Autodesk Inventor part; units mm, degrees
ref_plane "YZ Plane" through (0, 0, 0) normal (1, 0, 0) x (0, 1, 0)
ref_plane "XZ Plane" through (0, 0, 0) normal (0, 1, 0) x (-1, 0, 0)
ref_plane "XY Plane" through (0, 0, 0) normal (0, 0, 1) x (1, 0, 0)
sketch "スケッチ1" plane through (0, 0, 0) normal (0, 1, 0) x (-1, 0, 0)
  circle A0 centre (0, 0) radius 1.15
  circle A1 centre (0, 0) radius 2
  circle A2 centre (0, 0) radius 3.5
  line L0 (0, 0) -> (0, 3.5)
  line L1 (2, 0) -> (-2, 0)
  line L2 (2, 0) -> (2, -2.8723)
  line L3 (-2, 0) -> (-2, -2.8723)
  line L4 (0, 2) -> (3.5, 2)
  line L5 (3.5, 2) -> (3.5, 6)
  line L6 (3.5, 6) -> (0, 6)
  line L7 (0, 6) -> (0, 2)
  line L8 (0, 6) -> (3.5, 6)
  line L9 (3.5, 6) -> (3.5, 0)
  line L10 (3.5, 0) -> (0, 0)
  line L11 (0, 0) -> (0, 6)
  line L12 (0, 0) -> (0, -8)
  line L13 (0, 0) -> (3.5, 0)
  line L14 (3.5, 0) -> (3.5, -8)
  line L15 (3.5, -8) -> (0, -8)
  line L16 (0, -8) -> (0, 0)
  line L17 (2, -2.8723) -> (2, -8)
  line L18 (0, -8) -> (3.5, -4.5)
  line L19 (0, -8) -> (4.9497, -8) construction
  line L20 (0, 0) -> (3.5, 0)
  line L21 (3.5, 0) -> (3.5, -9)
  line L22 (3.5, -9) -> (0, -9)
  line L23 (0, -9) -> (0, 0)
  line L24 (0, 2) -> (4, 2)
  line L25 (4, 2) -> (4, 9)
  line L26 (4, 9) -> (0, 9)
  line L27 (0, 9) -> (0, 2)
  line L28 (0, 9) -> (4, 9)
  line L29 (4, 9) -> (4, -9)
  line L30 (4, -9) -> (0, -9)
  line L31 (0, -9) -> (0, 9)
  line L32 (0, 0) -> (2, 0)
  line L33 (2, 0) -> (2, -9)
  line L34 (2, -9) -> (0, -9)
  line L35 (0, -9) -> (0, 0)
  point P0 (2, -6)
  point P1 (0, -3.5)
  dimension "d0" = 2.3
  dimension "d1" = 4
  dimension "d2" = 7
  dimension "d3" = 3.5
  dimension "d4" = 4
  dimension "d5" = 8
  dimension "d6" = 45
  dimension "d40" = 9
  dimension "d41" = 4
  dimension "d42" = 7
extrude "押し出し1" add sketch "スケッチ1" along normal blind 3 contours A1 L3 A2 L0
extrude "押し出し2" add sketch "スケッチ1" along normal blind 4.5 contours L10 A2 L2 | A1 L4 A2 L10 | L0 A2 L4 | A2 L14 L18 L17 | A2 L4 L9 | L9 L24 L29 L30 L21 L14 | L7 L6 L5 L4 A2 | L18 L14 L15 L17 | L5 L6 L27 L26 L25 L24 | L15 L21 L22 L33
extrude "押し出し3" add sketch "スケッチ1" against normal blind 1 contours L1 A1 L12 A0 | A0 L0 A1 L1 | A0 L1 A1 L0 | L12 A1 L1 A0 | L2 A2 L12 A1 | L10 A2 L2 | A1 L4 A2 L10 | A1 L3 A2 L0 | L0 A2 L4 | L12 A2 L3 A1 | L17 L18 L12 A2 | A2 L14 L18 L17 | A2 L4 L9 | L9 L24 L29 L30 L21 L14 | L7 L6 L5 L4 A2 | L18 L14 L15 L17 | L17 L15 L18 | L5 L6 L27 L26 L25 L24 | L15 L33 L22 L23 | L15 L21 L22 L33
sketch "スケッチ4" plane through (0, 4.5, 0) normal (0, 1, 0) x (1, 0, 0)
  circle A0 centre (0, 0) radius 1.15
  circle A1 centre (0, 0) radius 2
  circle A2 centre (0, 0) radius 3.5
  line L0 (-4, 9) -> (-4, -9)
  line L1 (0, 0) -> (-4, 0)
  line L2 (-4, 0) -> (-4, -9)
  line L3 (-4, -9) -> (0, -9)
  line L4 (0, -9) -> (0, 0)
  line L5 (0, 0) -> (-4, 0)
  line L6 (-4, 0) -> (-4, 9)
  line L7 (-4, 9) -> (0, 9)
  line L8 (0, 9) -> (0, 0)
  point P0 (0, -3.5)
  point P1 (0, 3.5)
  dimension "d43" = 2.3
  dimension "d44" = 4
  dimension "d45" = 7
  dimension "d46" = 4
  dimension "d47" = 9
extrude "押し出し6" add sketch "スケッチ4" along normal blind 1 contours A0 L8 A1 L4 | A0 L1 A1 L8 | L4 A1 L1 A0 | L8 A2 L4 A1 | A1 L1 A2 L8 | L4 A2 L1 A1 | A2 L1 L0 L7 L8 | L4 L3 L0 L1 A2
sketch "スケッチ5" plane through (-4, -1, 9) normal (0, 0, 1) x (1, 0, 0)
  line L0 (4, 0) -> (4, 4)
  line L1 (4, 0) -> (0, 0)
  line L2 (0, 0) -> (0, 1)
  line L3 (0, 1) -> (4, 1)
  line L4 (4, 1) -> (4, 0)
  line L5 (4, 1) -> (2.5, 1)
  line L6 (2.5, 1) -> (2.5, 1.5)
  line L7 (2.5, 1.5) -> (4, 1.5)
  line L8 (4, 1.5) -> (4, 1)
  line L9 (4, 6.5) -> (0, 6.5)
  line L10 (0, 6.5) -> (2, 6.5)
  line L11 (2, 6.5) -> (2, 4.25)
  line L12 (2, 4.25) -> (0, 4.25)
  line L13 (0, 4.25) -> (0, 6.5)
  circle A0 centre (2, 4.25) radius 1.1
  dimension "d50" = 4
  dimension "d51" = 1
  dimension "d52" = 1.5
  dimension "d53" = 0.5
  dimension "d54" = 2
  dimension "d55" = 2.25
  dimension "d56" = 2.2
extrude "押し出し7" cut sketch "スケッチ5" against normal blind 7 contours A0 L12 L11 | L11 L12 A0
hole "穴2" at (-1.5, 0.5, 9) direction (0, 0, -1) diameter 1 end through all
chamfer "面取り1" distance 0.5 angle 45 3 edges at (0, -1, 6.25) (0, 5.5, 6.25) (-4, 5.5, 0)
chamfer "面取り2" distance 1.5 angle 45 1 edges at (-4, -1, 0)
sketch "スケッチ6" plane through (0, 0, -9) normal (0, 0, -1) x (-1, 0, 0)
  line L0 (0, 5.5) -> (4, 5.5)
  line L1 (4, 5.5) -> (4, -1)
  line L2 (4, -1) -> (0, -1)
  line L3 (0, -1) -> (0, 5.5)
  point P0 (0, 0)
  dimension "d72" = 4
  dimension "d73" = 6.5
extrude "押し出し8" cut sketch "スケッチ6" against normal blind 1
properties part number "rod6.2"
For this review, take the finished solid that the model builds, in its own axes (mm). A direction names the side the tool comes from. Coordinates: 2 decimals unless noted, no trailing zeros. Order: outer loops, then holes, each group sorted by start corner. A loop starts at its lowest first (then second) coordinate and runs counter-clockwise, first axis right, second up. Notation, with made-up numbers: (4, 57.5) -> (17, 57.5) arc R22 cw to (17, 65.5) -> close; hole circle Ø6 at (68, -35.75). An arc over 180 degrees is marked (long way). Return JSON: item names as keys, results as strings.
1. Machinability: for faces 5 (the flat face through (-4, 3, 1)), 6 (the cylindrical face through (0, 2, 2)), 7 (the flat face through (0, 5, -6)), 8 (the cylindrical face through (-0.95, 3.58, 5.55)), which of the approach directions +Z, -Z, +X, -X, +Y, -Y give a long, thin tool a straight path to every point of the face, cutting with its end or side? Answer none if there is none.
Answer block:
{"face 5": "+Z, -Z, -X, +Y, -Y", "face 6": "-Z", "face 7": "-Z, +X, +Y, -Y", "face 8": "+Z"}
2. We need section D-D on z = 2.25. Write out the cut boundary in (x, y), and give its area (3 significant figures).
Answer block:
{"outline": "(-4, 0.5) -> (-2.5, -1) -> (2.68, -1) -> (2.68, 3) -> (0, 3) -> (0, 4.5) -> (2.68, 4.5) -> (2.68, 5.5) -> (-3.5, 5.5) -> (-4, 5) -> close; hole circle Ø2.2 at (-2, 3.25); hole circle Ø1 at (-1.5, 0.5)", "area": "33.6 mm²"}
3. We need section A-A on x = 3.25. Write out the cut boundary in (y, z).
Answer block:
{"outline": "(-1, -1.3) -> (3, -1.3) -> (3, 1.3) -> (-1, 1.3) -> close; (4.5, -1.3) -> (5.5, -1.3) -> (5.5, 1.3) -> (4.5, 1.3) -> close"}
4. We need section B-B on z = -0.5. Write out the cut boundary in (x, y), and give its area (3 significant figures).
Answer block:
{"outline": "(-4, 0.5) -> (-2.5, -1) -> (-1.04, -1) -> (-1.04, 0) -> (-2, 0) -> (-2, 4.5) -> (-1.04, 4.5) -> (-1.04, 5.5) -> (-3.5, 5.5) -> (-4, 5) -> close; (1.04, -1) -> (3.46, -1) -> (3.46, 3) -> (2, 3) -> (2, 0) -> (1.04, 0) -> close; (1.04, 4.5) -> (3.46, 4.5) -> (3.46, 5.5) -> (1.04, 5.5) -> close", "area": "22.9 mm²"}
5. For pin 1 Ø1.8 at (x, z) = (0, 0) entering from +Y; pin 2 Ø1.1 at (x, y) = (-2, 3) entering from +Z; pin 3 Ø0.5 at (y, z) = (5, -5) entering from +X; pin 4 Ø3 at (y, z) = (1.5, -3.5) entering from +X, all flat-tipped, find the tip position at first contact; note any pin that passes through.
Answer block:
{"pin 1": "through", "pin 2": "z = 2", "pin 3": "x = 0", "pin 4": "x = 2.87"}
6. For line 1 (Y direction, x = 3, z = 1.5); line 2 (Y direction, x = -1.5, z = 5.25); line 3 (Y direction, x = -1.5, z = -1.75), list the stretches that pass through material, from the lowest coordinate up. Write a range as from..to.
Answer block:
{"line 1": "-1..3, 4.5..5.5", "line 2": "-1..0, 1..2.27, 4.23..5.5", "line 3": "-1..0, 4.5..5.5"}
7. The part is to be moulded in two halves that separate along Z. For faces 1 (the flat face through (-2, 1, 9)), 2 (the cylindrical face through (-0.91, 4.99, -0.7)), 3 (the cylindrical face through (0.91, -0.49, -0.7)), 4 (the flat face through (-2, 5.5, 0)), say which applies: +Z half, -Z half, draft (parallel to the pull), parting line (faces both ways), or undercut.
Answer block:
{"face 1": "+Z half", "face 2": "undercut", "face 3": "undercut", "face 4": "draft"}
8. We need section C-C on y = -0.25. Write out the cut boundary in (x, z).
Answer block:
{"outline": "(-3.25, -8) -> (0, -8) -> (0, -3.5) arc R3.5 ccw to (0, 3.5) -> (0, 9) -> (-3.25, 9) -> close; hole circle Ø2.3 at (0, 0)"}
